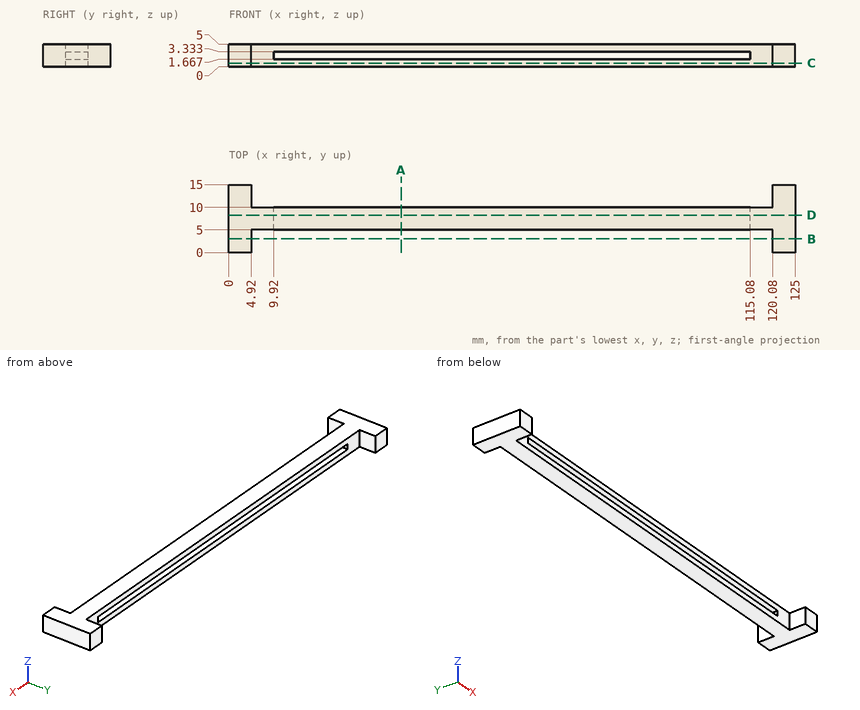
Source: three-view drawing plus pictorial views. Frame: mm from the lowest corner of the part. Give positions to 0.01 mm unless a question says otherwise; leave off trailing zeros. Order: outer loops, then holes, each group sorted by start corner. A loop starts at its lowest first (then second) coordinate and runs counter-clockwise, first axis right, second up.
1. Section A-A on x = 38. Return the cut outline in (y, z).
Derived:
outline: (5, 0) - (10, 0) - (10, 1.67) - (5, 1.67) - close; (5, 3.33) - (10, 3.33) - (10, 5) - (5, 5) - close
2. Section B-B on y = 3. Return the cut outline in (x, z).
Derived:
outline: (0, 0) - (4.92, 0) - (4.92, 5) - (0, 5) - close; (120.08, 0) - (125, 0) - (125, 5) - (120.08, 5) - close
3. Material intervals for L1, parallel to X at y = 9.5, z = 3; L2, parallel to X at y = 1.25, z = 1.75; L3, parallel to Z at x = 29.5, y = 8.25, sorted ascending.
Derived:
L1: x = 0 to 9.92, 115.08 to 125
L2: x = 0 to 4.92, 120.08 to 125
L3: z = 0 to 1.67, 3.33 to 5
4. Section D-D on y = 8.25. Return the cut outline in (x, z).
Derived:
outline: (0, 0) - (125, 0) - (125, 5) - (0, 5) - close; hole (9.92, 1.67) - (115.08, 1.67) - (115.08, 3.33) - (9.92, 3.33) - close
5. Pin query (flat end, axial travel): pin 1 (3 mm diameter, centred on x = 111.5, z = 3.5, fed in from +Y); pin 2 (1.5 mm diameter, centred on x = 78, z = 4, fed in from -Y); pin 3 (1.5 mm diameter, centred on x = 46.5, y = 8.5, fed in from -Z). Return the tip coordinate at first contact, or that it passes through.
Derived:
pin 1: stops at y = 10
pin 2: stops at y = 5
pin 3: stops at z = 0
6. Section C-C on z = 0.75. Return the cut outline in (x, y).
Derived:
outline: (0, 0) - (4.92, 0) - (4.92, 5) - (120.08, 5) - (120.08, 0) - (125, 0) - (125, 15) - (120.08, 15) - (120.08, 10) - (4.92, 10) - (4.92, 15) - (0, 15) - close
